```python
from build123d import *

# Parameters (mm, degrees)
SKETCH1_R           = 4.762500000000008
BOSS_EXTRUDE1_DEPTH = 38.1
SKETCH3_W           = 3.1750000000000043
SKETCH3_H           = 31.750000000000004
CUT_EXTRUDE1_DEPTH  = 12.7
SKETCH4_W           = 7.62
SKETCH4_H           = 6.350000000000001
SKETCH4_W_2         = 7.619999999999997
CUT_EXTRUDE2_DEPTH  = 60.05841387981902
SKETCH6_W           = 31.749999999999986
SKETCH6_H           = 31.750000000000004
CUT_EXTRUDE3_DEPTH  = 12.7
SKETCH7_W           = 38.1
SKETCH7_H           = 88.89999999999999
BOSS_EXTRUDE2_DEPTH = 3.175
FILLET1_R           = 2.54
FILLET2_R           = 12.7


with BuildPart() as part:
    # Sketch1 → Boss-Extrude1 (new body)
    # profile 1 of 3: a face of its own
    with BuildSketch(Plane(origin=(0, 0, 0), x_dir=(0, 0, -1), z_dir=(1, 0, 0))):
        Polygon((0, 0), (31.75, 3.89e-15), (31.749999999999993, 12.700000000000003), (0, 12.7), align=None)
    # profile 2 of 3: a face of its own
    with BuildSketch(Plane(origin=(0, 0, 0), x_dir=(0, 0, -1), z_dir=(1, 0, 0))):
        Polygon((28.575000000000003, 15.875000000000004), (3.1749999999999963, 15.875), (-3.1750000000000034, 15.875), (-3.1750000000000034, 12.7), (0, 12.7), (31.749999999999993, 12.700000000000003), (34.925, 12.700000000000005), (34.925, 15.875000000000004), align=None)
    # profile 3 of 3: a face of its own
    with BuildSketch(Plane(origin=(0, 0, 0), x_dir=(0, 0, -1), z_dir=(1, 0, 0))):
        with BuildLine():
            ThreePointArc((28.574999999999996, 31.75), (15.874999999999991, 44.45), (3.17499999999999, 31.749999999999996))
            Line((3.1749999999999936, 31.75), (3.174999999999996, 15.875))
            Line((3.1749999999999963, 15.875), (28.575000000000003, 15.875000000000004))
            Line((28.575, 15.875000000000004), (28.574999999999996, 31.75))
        make_face()
        with Locations(Location((15.874999999999996, 31.75, 0), (0, 0, 180))):
            Circle(SKETCH1_R, mode=Mode.SUBTRACT)
    extrude(amount=BOSS_EXTRUDE1_DEPTH)

    # Sketch3 → Cut-Extrude1 (cut)
    with BuildSketch(Plane.XZ):
        with Locations((1.5875000000000021, -15.875000000000002)):
            Rectangle(SKETCH3_W, SKETCH3_H)
        Polygon((34.92499999999999, 0), (34.92499999999999, -31.749999999999993), (38.1, -31.75), (38.1, 0), align=None)
    extrude(amount=-CUT_EXTRUDE1_DEPTH, mode=Mode.SUBTRACT)

    # Sketch4 → Cut-Extrude2 (cut, through all)
    with BuildSketch(Plane(origin=(0, 15.875, 1.45e-15), x_dir=(1, 0, 0), z_dir=(0, 1, 9e-17))):
        Polygon((15.240000000000002, 28.574999999999996), (7.620000000000001, 28.574999999999996), (7.620000000000005, -3.1750000000000043), (15.240000000000007, -3.175000000000002), align=None)
        Polygon((30.48, 28.574999999999996), (22.860000000000003, 28.574999999999996), (22.860000000000007, -3.1750000000000043), (30.480000000000008, -3.175000000000002), align=None)
        with Locations((11.43, 31.749999999999996)):
            Rectangle(SKETCH4_W, SKETCH4_H)
        with Locations((26.67, 31.749999999999996)):
            Rectangle(SKETCH4_W_2, SKETCH4_H)
    extrude(amount=CUT_EXTRUDE2_DEPTH, mode=Mode.SUBTRACT)

    # Sketch6 → Cut-Extrude3 (cut)
    with BuildSketch(Plane.XZ):
        with Locations((19.049999999999997, -15.875000000000002)):
            Rectangle(SKETCH6_W, SKETCH6_H)
    extrude(amount=-CUT_EXTRUDE3_DEPTH, mode=Mode.SUBTRACT)

    # Sketch7 → Boss-Extrude2 (add)
    with BuildSketch(Plane.XZ.offset(-12.7)):
        with Locations((19.05, -15.875)):
            Rectangle(SKETCH7_W, SKETCH7_H)
    extrude(amount=-BOSS_EXTRUDE2_DEPTH)

    # Fillet1
    fillet1_edges = [part.edges().sort_by_distance(p)[0] for p in [
        (30.480000000000004, 15.875000000000002, -15.875),
        (22.860000000000003, 15.875000000000002, -15.875),
        (15.240000000000004, 15.875000000000002, -15.875),
        (7.620000000000003, 15.875000000000002, -15.875),
    ]]
    fillet(fillet1_edges, radius=FILLET1_R)

    # Fillet2
    fillet2_edges = [part.edges().sort_by_distance(p)[0] for p in [
        (33.02, 15.875, -3.1749999999999963),
    ]]
    fillet(fillet2_edges, radius=FILLET2_R)
    fillet2_2_edges = [part.edges().sort_by_distance(p)[0] for p in [
        (5.080000000000002, 15.875, -3.1749999999999963),
    ]]
    fillet(fillet2_2_edges, radius=FILLET2_R)
    fillet2_3_edges = [part.edges().sort_by_distance(p)[0] for p in [
        (5.08, 15.875000000000004, -28.575000000000003),
    ]]
    fillet(fillet2_3_edges, radius=FILLET2_R)
    fillet2_4_edges = [part.edges().sort_by_distance(p)[0] for p in [
        (33.02, 15.875000000000004, -28.575000000000003),
    ]]
    fillet(fillet2_4_edges, radius=FILLET2_R)
    fillet2_5_edges = [part.edges().sort_by_distance(p)[0] for p in [
        (19.050000000000008, 15.875, -3.174999999999996),
    ]]
    fillet(fillet2_5_edges, radius=FILLET2_R)
    fillet2_6_edges = [part.edges().sort_by_distance(p)[0] for p in [
        (19.050000000000004, 15.875000000000002, -28.575),
    ]]
    fillet(fillet2_6_edges, radius=FILLET2_R)


solid = part.part
```
The model under review builds one solid part; all positions refer to its coordinate system, in mm. A direction names the side the tool comes from. Coordinates: 2 decimals unless noted, no trailing zeros. Loops run counter-clockwise (first coordinate to the right, second up) from the corner with the lowest first, then second, coordinate; pieces in that order, holes last. Notation, with made-up numbers: (2, 74.5) -> (18, 74.5) arc R19 ccw to (18, 90.5) -> close; hole circle Ø4 at (43.5, 28). An arc over 180 degrees is marked (long way). Answer as CSV lines item,"result".
Item 1: For L1, parallel to X at y = 19.5, z = -16.5; L2, parallel to Z at x = 36.5, y = 31.75 (1 decimal); L3, parallel to Y at x = 24.5, z = 9.5, list the stretches that pass through material, from the lowest coordinate up.
Results below:
L1,"x = 0 to 7.62, 15.24 to 22.86, 30.48 to 38.1"
L2,"z = -28.6 to -20.6, -11.1 to -3.2"
L3,"y = 12.7 to 15.88"
Item 2: Take a section at C-C, the plane y = 37.5. State the section outline as (x, z) points, and give its area (3 significant figures).
Results below:
outline,"(0, -27.2) -> (7.62, -27.2) -> (7.62, -4.55) -> (0, -4.55) -> close; (15.24, -27.2) -> (22.86, -27.2) -> (22.86, -4.55) -> (15.24, -4.55) -> close; (30.48, -27.2) -> (38.1, -27.2) -> (38.1, -4.55) -> (30.48, -4.55) -> close"
area,"518 mm2"
Item 3: Draft analysis for pull direction Y (two halves, no side actions). For faces 5 (the cylindrical face through (14.476, 16.599, -16.231)), 6 (the flat face through (34, 30, -3.175)), 7 (the cylindrical face through (3.757, 31.541, -20.633)), state which applies: +Y half, -Y half, draft (parallel to the pull), parting line (faces both ways), or undercut.
Results below:
face 5,"+Y half"
face 6,"draft"
face 7,"undercut"
Item 4: Insertion check: pin 1 (7.5 mm diameter, centred on y = 31.75, z = -15.875, fed in from -X); pin 2 (2.5 mm diameter, centred on x = 36, y = 30.5, fed in from +Z) (3 decimals); pin 3 (1.5 mm diameter, centred on x = 20.5, y = 26.5, fed in from +Z); pin 4 (3.5 mm diameter, centred on x = 5.5, y = 31, fed in from -Z) (3 decimals). Each pin has a flat end and moves straight along its axis. Give the tip position at first contact, or say it passes through.
Results below:
pin 1,"passes through"
pin 2,"stops at z = -3.175"
pin 3,"stops at z = -2.86"
pin 4,"stops at z = -28.575"
Item 5: Machinability: for faces 1 (the cylindrical face through (18.96, 19.5, 0.64)), 2 (the cylindrical face through (8.344, 16.639, -15.519)), 3 (the flat face through (19, 30, -28.575)), 4 (the flat face through (10.32, 15.875, -15.25)), which of the approach directions +Z, -Z, +X, -X, +Y, -Y give a long, thin tool a straight path to every point of the face, cutting with its end or side? Answer none if there is none.
Results below:
face 1,"+Z, +X, -X, +Y"
face 2,"+Z, -Z, +Y"
face 3,"-Z, +X, -X, +Y"
face 4,"+Y"
Item 6: Take a section at D-D, the plane z = -22.5. State the section outline as (x, y) points (3 decimals).
Results below:
outline,"(0, 12.7) -> (38.1, 12.7) -> (38.1, 42.585) -> (30.48, 42.585) -> (30.48, 18.415) arc R2.54 cw to (27.94, 15.875) -> (25.4, 15.875) arc R2.54 cw to (22.86, 18.415) -> (22.86, 42.585) -> (15.24, 42.585) -> (15.24, 18.415) arc R2.54 cw to (12.7, 15.875) -> (10.16, 15.875) arc R2.54 cw to (7.62, 18.415) -> (7.62, 42.585) -> (0, 42.585) -> close"
Item 7: Take a section at A-A, the plane y = 33.5. State the section outline as (x, z) points, and give its area (3 significant figures).
Results below:
outline,"(0, -28.45) -> (7.62, -28.45) -> (7.62, -20.3) -> (0, -20.3) -> close; (0, -11.45) -> (7.62, -11.45) -> (7.62, -3.3) -> (0, -3.3) -> close; (15.24, -28.45) -> (22.86, -28.45) -> (22.86, -20.3) -> (15.24, -20.3) -> close; (15.24, -11.45) -> (22.86, -11.45) -> (22.86, -3.3) -> (15.24, -3.3) -> close; (30.48, -28.45) -> (38.1, -28.45) -> (38.1, -20.3) -> (30.48, -20.3) -> close; (30.48, -11.45) -> (38.1, -11.45) -> (38.1, -3.3) -> (30.48, -3.3) -> close"
area,"373 mm2"
